```python
from build123d import *

# Parameters (mm, degrees)
BOSS_EXTRU_1_DEPTH      = 5
ESQUISSE9_W             = 5
ESQUISSE9_H             = 5
BOSS_EXTRU_3_DEPTH      = 40
ESQUISSE12_R            = 1.048820472
ENL_V_MAT_EXTRU_3_DEPTH = 40
CONG_3_R                = 3
CONG_4_R                = 3


with BuildPart() as part:
    # Esquisse1 → Boss.-Extru.1 (new body)
    with BuildSketch(Plane.XY):
        with BuildLine():
            Line((26.025021052, -0.447992933), (-24.829805977, 87.508811894))
            Line((-24.829805977, 87.508811894), (-24.829805977, 1.293439737))
            ThreePointArc((-24.829805977, 1.293439737), (1.080284786, 14.518282983), (26.025021052, -0.447992933))
        make_face()
    extrude(amount=BOSS_EXTRU_1_DEPTH)

    # Esquisse9 → Boss.-Extru.3 (add)
    with BuildSketch(Plane(origin=(0, 47.4898845, 0), x_dir=(1, 0, 0), z_dir=(0, 1, 0))):
        with Locations((-27.329805977, -2.5)):
            Rectangle(ESQUISSE9_W, ESQUISSE9_H)
    extrude(amount=-BOSS_EXTRU_3_DEPTH)

    # Esquisse12 → Enlèv. mat.-Extru.3 (cut)
    with BuildSketch(Plane(origin=(0, 47.4898845, 0), x_dir=(1, 0, 0), z_dir=(0, 1, 0))):
        with Locations(Location((-27.329805977, -2.5, 0), (0, 0, 270))):
            Circle(ESQUISSE12_R)
    extrude(amount=-ENL_V_MAT_EXTRU_3_DEPTH, mode=Mode.SUBTRACT)

    # Congé3
    cong_3_edges = [part.edges().sort_by_distance(p)[0] for p in [
        (-29.829805977, 27.4898845, 5),
    ]]
    fillet(cong_3_edges, radius=CONG_3_R)

    # Congé4
    # the kernel refuses this fillet: 3 mm, written as the material it takes off along each edge
    with BuildSketch(Plane(origin=(-29.829805977, 54.560952312, 0), x_dir=(0, 0, 1), z_dir=(0, -1, 0))) as cong_4_piece_1:
        with BuildLine():
            CenterArc((3, -2.828427125), CONG_4_R, 109.471220634, 70.528779366)
            Line((0, -2.828427125), (-0.06, -2.828427125))
            Line((-0.06, -2.828427125), (-0.06, 0))
            Line((-0.06, 0), (0, 0.06))
            ThreePointArc((0, 0.06), (1, 0.06), (1.98, 0.056568542))
            Line((1.98, 0.056568542), (2, 0))
        make_face()
    extrude(amount=54.142135624, mode=Mode.SUBTRACT)


solid = part.part
```
Can you work these out from the model? Positions are in its coordinate system, mm. A direction names the side the tool comes from. Give positions to 0.01 mm unless a question says otherwise; leave off trailing zeros. Loops run counter-clockwise (first coordinate to the right, second up) from the corner with the lowest first, then second, coordinate; pieces in that order, holes last. Notation, with made-up numbers: M -35,3.5 L -20,3.5 A33 cw -20,38.5 Z; hole C 38.25,75 d7. An arc over 180 degrees is marked long. Answer in a Markdown table with one row per item.
1. If I drill on line 1 along X through (y, z) = (11, 2.75); line 2 along Y through (x, z) = (-25, 1.9); line 3 along X through (y, z) = (28, 2.3), over which ranges is the centre line in solid material (lowest first)?
Taken from the geometry:
| item | result |
|---|---|
| line 1 | x = -29.73 to -28.35, -26.31 to -14.08, 14.18 to 19.41 |
| line 2 | y = 7.49 to 47.49 |
| line 3 | x = -29.81 to -28.36, -26.3 to 9.58 |
2. Suppose I cut it at D-D on y = 69.5. Write out the boundary of the cut face in (x, z), plus the area to 3 significant figures.
Taken from the geometry:
| item | result |
|---|---|
| outline | M -24.83,0 L -14.42,0 L -14.42,5 L -24.83,5 Z |
| area | 52.1 mm² |
3. For pin 1 Ø1.5 at (x, z) = (-27.5, 3.5) entering from -Y; pin 2 Ø1.5 at (x, z) = (-27, 1.5) entering from +Y; pin 3 Ø2.5 at (y, z) = (5, 3.5) entering from -X, each with a flat end and sliding along its axis, tell me the tip position at first contact or that it passes through.
Taken from the geometry:
| item | result |
|---|---|
| pin 1 | stops at y = 7.49 |
| pin 2 | stops at y = 47.49 |
| pin 3 | stops at x = -24.83 |
4. Thinking about a two-plate mould opening in Z: for faces 1 (the cylindrical face through (-26.29, 27.77, 2.36)), 2 (the flat face through (-26, 7.49, 2)), 3 (the cylindrical face through (-28.8, 27.8, 0.6)), 4 (the flat face through (-13, 34, 5)), which applies, released by +Z, released by -Z, zero draft, split by the parting line, or undercut?
Taken from the geometry:
| item | result |
|---|---|
| face 1 | undercut |
| face 2 | zero draft |
| face 3 | released by -Z |
| face 4 | released by +Z |
5. Which directions (+Z, -Z, +X, -X, +Y, -Y) give clear straight access to the entire face, cutting with the end or side of a thin tool? Please do faces 5 (the cylindrical face through (0.66, 14.53, 2.46)), 6 (the flat face through (-24.83, 4, 2)), 7 (the flat face through (-24.83, 68, 2)).
Taken from the geometry:
| item | result |
|---|---|
| face 5 | +Z, -Z, -Y |
| face 6 | +Z, -Z, -X, -Y |
| face 7 | +Z, -Z, -X, +Y |
6. Suppose I cut it at C-C on y = 46. Write out the boundary of the cut face in (x, z), plus the area to 3 significant figures.
Taken from the geometry:
| item | result |
|---|---|
| outline | M -29.83,2 A3 ccw -27,0 L -0.83,0 L -0.83,5 L -26.83,5 A3 ccw Z; hole C -27.33,2.5 d2.1 |
| area | 138 mm² |
7. Suppose I cut it at A-A on y = 28. Write out the boundary of the cut face in (x, z).
Taken from the geometry:
| item | result |
|---|---|
| outline | M -29.83,2 A3 ccw -27,0 L 9.58,0 L 9.58,5 L -26.83,5 A3 ccw Z; hole C -27.33,2.5 d2.1 |
8. Suppose I cut it at B-B on x = 7.5. Write out the boundary of the cut face in (y, z).
Taken from the geometry:
| item | result |
|---|---|
| outline | M 13.6,0 L 31.59,0 L 31.59,5 L 13.6,5 Z |
